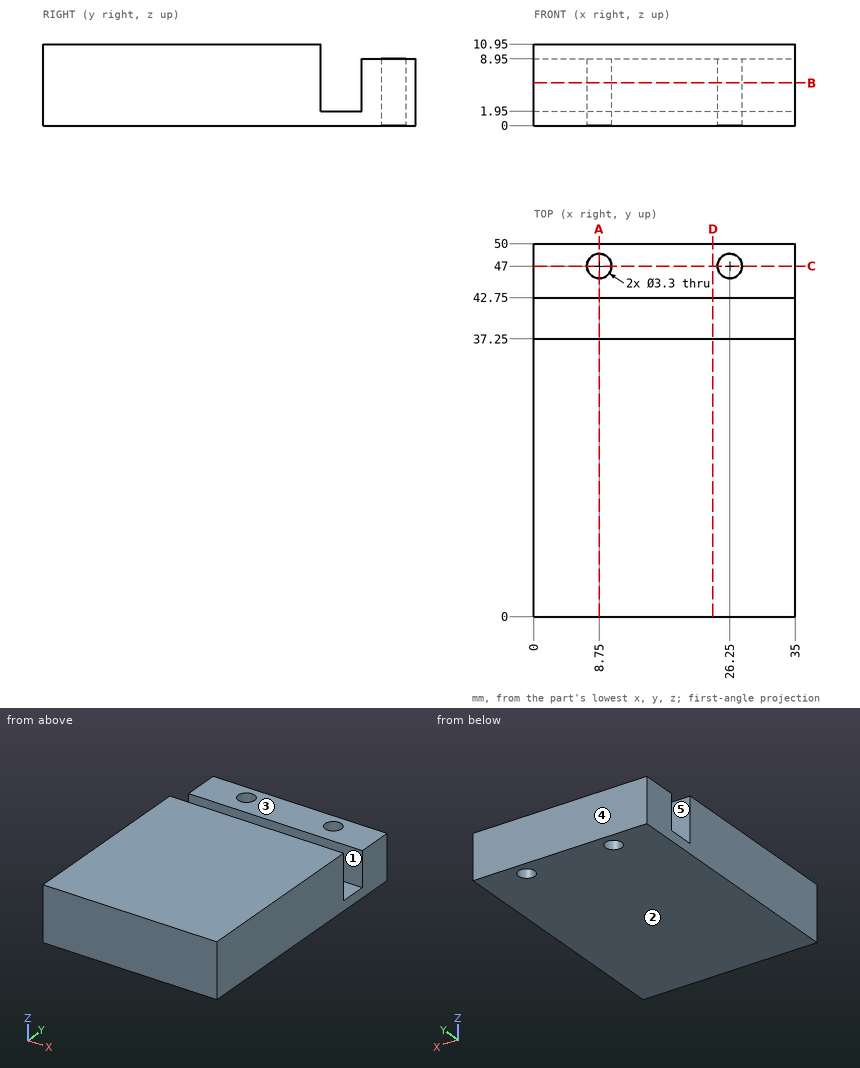
Could you check a few things on this drawing? It's one solid part, dimensions in mm from its lowest x, y, z. A direction names the side the tool comes from. Coordinates: 2 decimals unless noted, no trailing zeros. Write each loop counter-clockwise with the first axis right and the second up, starting at its lowest first coordinate (ties: lowest second). Pieces come first, ordered by that corner, then holes. Notation, with made-up numbers: (47, -10) - (71, -10) arc R20 ccw to (71, 27) - close; hole circle Ø9 at (51, 73.5). An arc over 180 degrees is marked (long way). Return JSON: item names as keys, results as strings. Group by question number.
Item 1: If we section it at C-C (y = 47): Write out the boundary of the cut face in (x, z).
Item 2: If we section it at B-B (z = 5.75): Write out the boundary of the cut face in (x, y), then the cut area to 3 significant figures.
Item 3: We'd pull the mould along Y, two halves only. Please class the marked faces 3, 4 and 5: pulls with the +Y half, pulls with the -Y half, needs draft (parallel to the pull), parting line crosses it, or undercut.
Item 4: Please list where these lines run through material, in increasing order: probe 1 along X at (y, z) = (47, 7); probe 2 along Y at (x, z) = (26.25, 6.5); probe 3 along Y at (x, z) = (5, 5.5).
Item 5: I'm going to push a flat-ended pin straight in: pin 1 Ø4.5 at (x, y) = (26.25, 47) entering from +Z. Where does the tip first touch, or does it pass through?
Item 6: If we section it at D-D (x = 24): Write out the boundary of the cut face in (y, z), then the cut area to 4 significant figures.
Item 7: Which directions (+Z, -Z, +X, -X, +Y, -Y) give clear straight access to the entire face, cutting with the end or side of a thin tool? Please do the marked faces 1 and 2.
Item 8: If we section it at A-A (x = 8.75): Write out the boundary of the cut face in (y, z), then the cut area to 3 significant figures.
Return value:
{
 "1": {"outline": "(0, 0) - (7.1, 0) - (7.1, 8.95) - (0, 8.95) - close; (10.4, 0) - (24.6, 0) - (24.6, 8.95) - (10.4, 8.95) - close; (27.9, 0) - (35, 0) - (35, 8.95) - (27.9, 8.95) - close"},
 "2": {"outline": "(0, 0) - (35, 0) - (35, 37.25) - (0, 37.25) - close; (0, 42.75) - (35, 42.75) - (35, 50) - (0, 50) - close; hole circle Ø3.3 at (8.75, 47); hole circle Ø3.3 at (26.25, 47)", "area": "1,540 mm^2"},
 "3": {"face 3": "needs draft", "face 4": "pulls with the +Y half", "face 5": "undercut"},
 "4": {"probe 1": "x = 0 to 7.1, 10.4 to 24.6, 27.9 to 35", "probe 2": "y = 0 to 37.25, 42.75 to 45.35, 48.65 to 50", "probe 3": "y = 0 to 37.25, 42.75 to 50"},
 "5": {"pin 1": "stops at z = 8.95"},
 "6": {"outline": "(0, 0) - (50, 0) - (50, 8.95) - (42.75, 8.95) - (42.75, 1.95) - (37.25, 1.95) - (37.25, 10.95) - (0, 10.95) - close", "area": "483.5 mm^2"},
 "7": {"face 1": "+Z, +X, -X", "face 2": "-Z, +X, -X, +Y, -Y"},
 "8": {"outline": "(0, 0) - (45.35, 0) - (45.35, 8.95) - (42.75, 8.95) - (42.75, 1.95) - (37.25, 1.95) - (37.25, 10.95) - (0, 10.95) - close; (48.65, 0) - (50, 0) - (50, 8.95) - (48.65, 8.95) - close", "area": "454 mm^2"}
}
